from build123d import *

# Parameters (mm, degrees)
SKICA1_W            = 150
SKICA1_H            = 80
VYSUNOUT1_DEPTH     = 3
SKICA2_RX           = 12.5
SKICA2_RY           = 5
VYSUNOUT2_DEPTH     = 10
LINPOLE1_COUNT      = 9
LINPOLE1_PITCH      = 15
LINPOLE1_COUNT_DIR2 = 2
LINPOLE1_PITCH_DIR2 = 40


with BuildPart() as part:
    # Skica1 → Vysunout1 (new body)
    with BuildSketch(Plane.XY):
        with Locations((75, 40)):
            Rectangle(SKICA1_W, SKICA1_H)
    extrude(amount=VYSUNOUT1_DEPTH)

    # Skica2 → Vysunout2 (add)
    with BuildSketch(Plane.XY.offset(3)):
        with Locations(Location((15, 60), (0, 0, 90))):
            Ellipse(SKICA2_RX, SKICA2_RY)
    vysunout2 = extrude(amount=VYSUNOUT2_DEPTH)

    # LinPole1: Vysunout2 9 × 2
    with Locations(*[(i * LINPOLE1_PITCH, -j * LINPOLE1_PITCH_DIR2, 0) for i in range(LINPOLE1_COUNT) for j in range(LINPOLE1_COUNT_DIR2) if (i, j) != (0, 0)]):
        add(vysunout2)


solid = part.part
The listing builds one solid part. Answer for the finished solid, in the listing's coordinates (mm). Round coordinates to 2 decimals unless told otherwise and drop trailing zeros. Write each question's results on one line, items separated by ' | '. Start each with the question number.
1) Each of these flat-tipped pins is pushed along its axis until it touches: pin 1 (1 mm diameter, centred on y = 35, z = 2, fed in from -X); pin 2 (1.5 mm diameter, centred on y = 13, z = 11.5, fed in from +X); pin 3 (1 mm diameter, centred on x = 18, z = 7, fed in from -Y); pin 4 (5 mm diameter, centred on y = 47, z = 7, fed in from -X). Where does it stop, or does it pass through?
2) Find section A-A on z = 8.5. Count the separate pieces of the cut face and the enclosed holes in it, plus the area to 3 significant figures.
3) Straight lines are drawn through the part: probe 1 along Z at (x, y) = (124.5, 53.5); probe 2 along Y at (x, z) = (17.5, 11.25); probe 3 along Y at (x, z) = (108, 3.75). For each, find the intervals that lie inside material, in ascending order.
4) Determine the mould class of faces 1 (the flat face through (74, 41, 3)), 2 (the flat face through (0, 39, 1)), 3 (the flat face through (105, 60, 13)) for opening direction X: pulls with the +X half, pulls with the -X half, needs draft (parallel to the pull), parting line crosses it, or undercut.
Final values:
1) pin 1: x = 0 | pin 2: x = 139.33 | pin 3: y = 9.17 | pin 4: x = 12.29
2) separate pieces: 18 | enclosed holes: 0 | area: 3,530 mm²
3) probe 1: 0 to 3 | probe 2: 9.17 to 30.83, 49.17 to 70.83 | probe 3: 10 to 30, 50 to 70
4) face 1: undercut | face 2: pulls with the -X half | face 3: needs draft
